Geometry: final body of the model. Coordinates: model frame, mm. Face numbers are marked on the shaded views. A direction names the side the tool comes from. Give positions to 0.01 mm unless a question says otherwise; leave off trailing zeros. Write each loop counter-clockwise with the first axis right and the second up, starting at its lowest first coordinate (ties: lowest second). Pieces come first, ordered by that corner, then holes. Notation, with made-up numbers: (-8, -9) -> (46, -9) arc R19 ccw to (46, 7) -> close; hole circle Ø3 at (45.25, -27.5). An arc over 180 degrees is marked (long way). Use CSV: the item, a comma, the result in double quotes. Start each with the question number.
1) Material intervals for line 1 (Z direction, x = 13, y = 46.5) (3 decimals); line 2 (X direction, y = 27.5, z = 8.5) (3 decimals), sorted ascending. Write a range as [from, to].
2) Section B-B (z = -52.5). Output: boundary loops of the cut face in (x, y) (3 decimals).
3) Section A-A (y = 53). Output: boundary loops of the cut face in (x, z) (3 decimals), plus the area to 3 significant figures.
4) Set-up query: the marked faces 1 and 2. Return all of +Z, -Z, +X, -X, +Y, -Y with unobstructed straight access to the full face (end or side cutting, diameter ignored); none if empty.
5) Contact query for flat-ended pins moving along their axis: P1, Ø8, axis at x = -5.5, z = -65.5, coming from the +Y side (3 decimals); P2, Ø3.5, axis at x = -33.5, z = -35, coming from the +Y side (3 decimals). Output: stop coordinate, or through.
6) Section C-C (x = 5). Output: boundary loops of the cut face in (y, z) (3 decimals), plus the area to 3 significant figures.
7) Draft query along X for the marked faces 3, 4 and 5. Return one class per face: pulls with the +X half, pulls with the -X half, needs draft (parallel to the pull), parting line crosses it, or undercut.
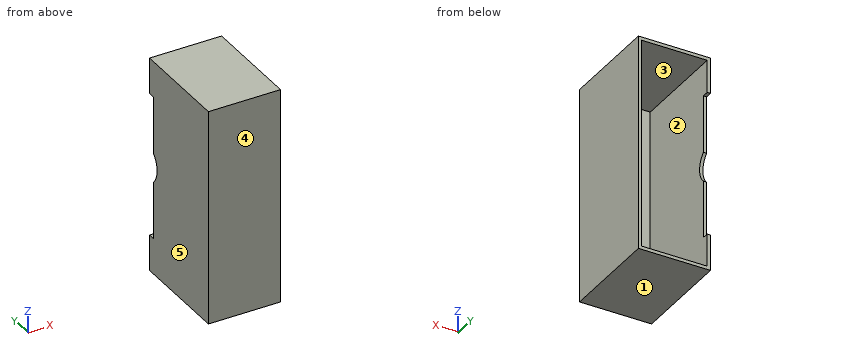
```python
from build123d import *

# Parameters (mm, degrees)
SKETCH1_W           = 69.85
SKETCH1_H           = 209.55
BOSS_EXTRUDE1_DEPTH = 98.425
SKETCH2_W           = 63.5
SKETCH2_H           = 203.2
CUT_EXTRUDE1_DEPTH  = 95.25
CUT_EXTRUDE2_DEPTH  = 3.175


with BuildPart() as part:
    # Sketch1 → Boss-Extrude1 (new body)
    with BuildSketch(Plane(origin=(0, 0, 0), x_dir=(1, 0, 0), z_dir=(0, 1, 0))):
        Rectangle(SKETCH1_W, SKETCH1_H)
    extrude(amount=BOSS_EXTRUDE1_DEPTH)

    # Sketch2 → Cut-Extrude1 (cut)
    with BuildSketch(Plane(origin=(0, 98.425, 0), x_dir=(1, 0, 0), z_dir=(0, 1, 0))):
        Rectangle(SKETCH2_W, SKETCH2_H)
    extrude(amount=-CUT_EXTRUDE1_DEPTH, mode=Mode.SUBTRACT)

    # Sketch3 → Cut-Extrude2 (cut)
    with BuildSketch(Plane.ZY.offset(34.925)):
        with BuildLine():
            Line((-69.896994772, 98.425), (-69.896994772, 178.106960935))
            Line((-69.896994772, 178.106960935), (69.896994772, 178.106960935))
            Line((69.896994772, 178.106960935), (69.896994772, 98.425))
            Line((69.896994772, 98.425), (69.896994772, 92.075))
            Line((69.896994772, 92.075), (14.246026429, 92.075))
            ThreePointArc((14.246026429, 92.075), (0, 85.672261798), (-14.246026429, 92.075))
            Line((-14.246026429, 92.075), (-69.896994772, 92.075))
            Line((-69.896994772, 92.075), (-69.896994772, 98.425))
        make_face()
    extrude(amount=-CUT_EXTRUDE2_DEPTH, mode=Mode.SUBTRACT)


solid = part.part
```
Answers follow:
1,line 1,"z = [-104.775, -101.6], [101.6, 104.775]"
1,line 2,"x = [-34.925, -31.75], [31.75, 34.925]"
2,outline,"(-34.925, 0) -> (34.925, 0) -> (34.925, 98.425) -> (31.75, 98.425) -> (31.75, 3.175) -> (-31.75, 3.175) -> (-31.75, 92.075) -> (-34.925, 92.075) -> close"
3,outline,"(-34.925, -104.775) -> (34.925, -104.775) -> (34.925, 104.775) -> (-34.925, 104.775) -> close; hole (-31.75, -101.6) -> (31.75, -101.6) -> (31.75, 101.6) -> (-31.75, 101.6) -> close"
3,area,"1,730 mm^2"
4,face 1,"-Z, +X, -X, +Y, -Y"
4,face 2,"+Y"
5,P1,"stops at y = 3.175"
5,P2,"stops at y = 92.075"
6,outline,"(0, -104.775) -> (98.425, -104.775) -> (98.425, -101.6) -> (3.175, -101.6) -> (3.175, 101.6) -> (98.425, 101.6) -> (98.425, 104.775) -> (0, 104.775) -> close"
6,area,"1,270 mm^2"
7,face 3,"undercut"
7,face 4,"needs draft"
7,face 5,"pulls with the -X half"
